Verification items for this drawing (mm, ordinates from the low corner). Round coordinates to 2 decimals unless told otherwise and drop trailing zeros. Order: outer loops, then holes, each group sorted by start corner. A loop starts at its lowest first (then second) coordinate and runs counter-clockwise, first axis right, second up. Notation, with made-up numbers: M -27,24 L -16,24 A30 ccw -16,63 Z; hole C -30.75,68 d8. An arc over 180 degrees is marked long. Use CSV: the item, a comma, the result in double quotes. Start each with the question number.
Q1. Sectioned sample at A-A (x = 21.5). State how many separate pieces and enclosed holes the cut face has, and give its area (3 significant figures).
Q2. Scan lines: line 1 (X direction, y = 7, z = 125.5) (1 decimal); line 2 (Z direction, x = 18, y = 4.25) (1 decimal); line 3 (Z direction, x = 52.5, y = 4.25). Record each from-to range of solid material in increasing order.
Q3. Sectioned sample at D-D (z = 116.5). Enter the section's corners in (x, y) (1 decimal), and give its area (3 significant figures).
Q4. Gauge pin test, flat ends, axial feed: pin 1 Ø3 at (y, z) = (6.5, 19) entering from +X; pin 2 Ø2.5 at (x, z) = (53.57, 125.17) entering from -Y; pin 3 Ø3.5 at (y, z) = (4.76, 57.15) entering from +X (1 decimal); pin 4 Ø5 at (y, z) = (4.76, 19.05) entering from -X. Record the tip position at first contact, or that the pin passes through.
Q5. Mould release check, pull along X, two halves, no side actions. Record for the marked faces 1, 2, 3 and 4: +X half, -X half, draft (parallel to the pull), parting line (faces both ways), or undercut.
Q6. Sectioned sample at B-B (z = 101.6). Enter the section's corners in (x, y) (1 decimal).
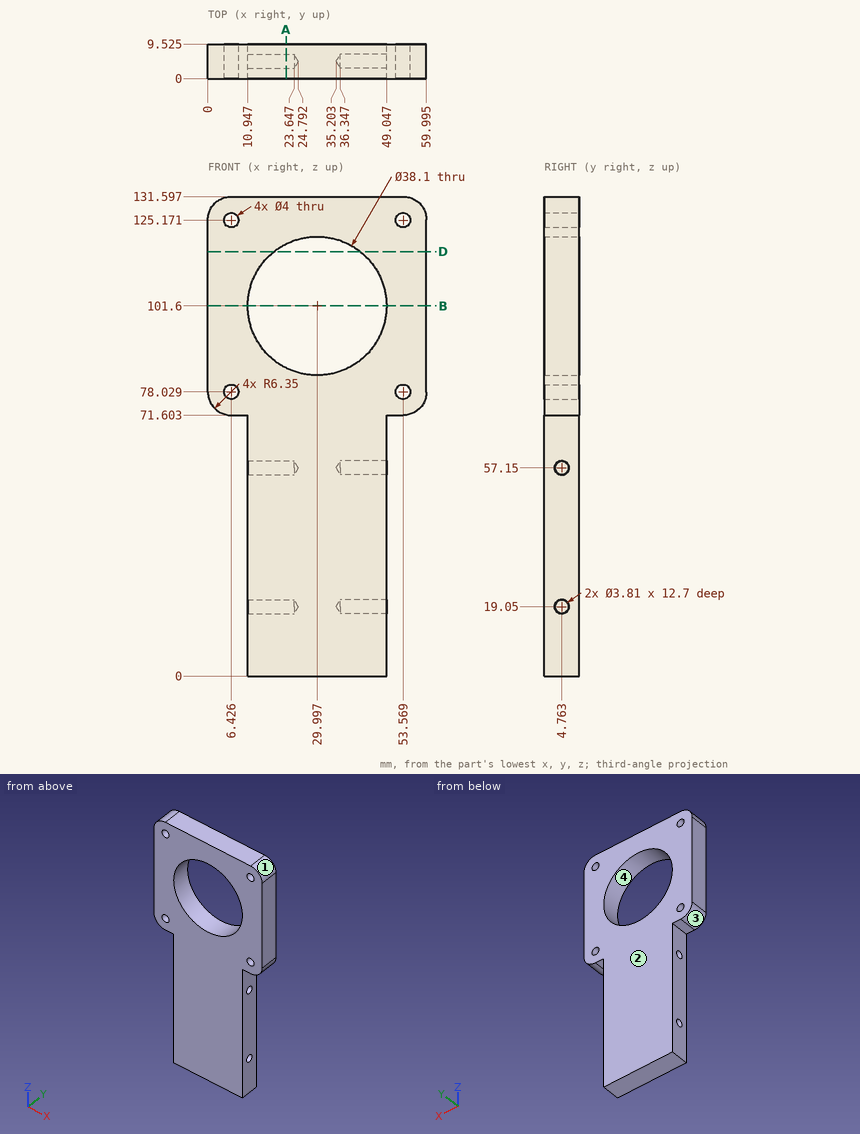
Verdict:
1,separate pieces,"2"
1,enclosed holes,"2"
1,area,"906 mm²"
2,line 1,"x = 0 to 4.5, 8.4 to 51.6, 55.5 to 60"
2,line 2,"z = 0 to 17.2, 20.9 to 55.3, 59 to 86.8, 116.4 to 131.6"
2,line 3,"z = 71.6 to 76.34, 79.72 to 123.48, 126.86 to 131.6"
3,outline,"M 0,0 L 18.1,0 L 18.1,9.5 L 0,9.5 Z; M 41.9,0 L 60,0 L 60,9.5 L 41.9,9.5 Z"
3,area,"345 mm²"
4,pin 1,"stops at x = 49.05"
4,pin 2,"passes through"
4,pin 3,"stops at x = 36.3"
4,pin 4,"stops at x = 10.95"
5,face 1,"+X half"
5,face 2,"draft"
5,face 3,"-X half"
5,face 4,"undercut"
6,outline,"M 0,0 L 10.9,0 L 10.9,9.5 L 0,9.5 Z; M 49,0 L 60,0 L 60,9.5 L 49,9.5 Z"
